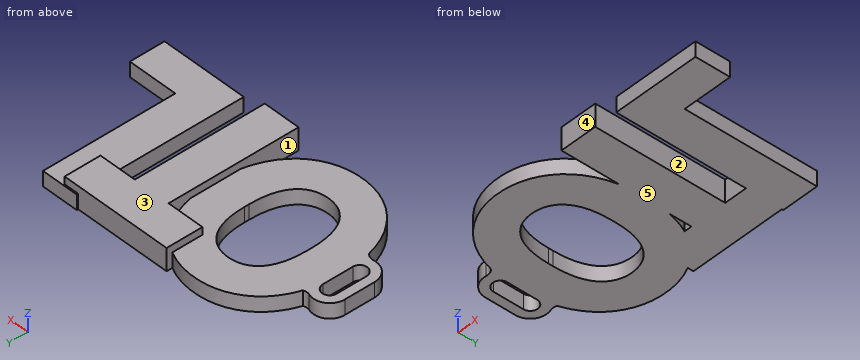
from build123d import *

# Parameters (mm, degrees)
PAD_DEPTH    = 2
PAD001_DEPTH = 3
PAD002_DEPTH = 2
PAD003_DEPTH = 2


with BuildPart() as part:
    # Sketch001 → Pad (new body)
    with BuildSketch(Plane.XY):
        with BuildLine():
            add(Edge.make_bspline(
                [(11.345455, -0.198864), (16.382955, -0.198864), (20.826136, 3.529545), (20.826136, 10.782955)],
                knots=[0, 0, 0, 0, 1, 1, 1, 1], degree=3))
            Line((20.826136, 10.782955), (20.826136, 11.417045))
            add(Edge.make_bspline(
                [(20.826136, 11.417045), (20.826136, 18.670455), (16.382955, 22.4), (11.345455, 22.4)],
                knots=[0, 0, 0, 0, 1, 1, 1, 1], degree=3))
            add(Edge.make_bspline(
                [(11.345455, 22.4), (6.306818, 22.4), (1.903409, 18.670455), (1.903409, 11.417045)],
                knots=[0, 0, 0, 0, 1, 1, 1, 1], degree=3))
            Line((1.903409, 11.417045), (1.903409, 10.782955))
            add(Edge.make_bspline(
                [(1.903409, 10.782955), (1.903409, 3.529545), (6.306818, -0.198864), (11.345455, -0.198864)],
                knots=[0, 0, 0, 0, 1, 1, 1, 1], degree=3))
        make_face()
        with BuildLine():
            add(Edge.make_bspline(
                [(11.345455, 4.363636), (9.004545, 4.363636), (6.782955, 5.948864), (6.782955, 10.782955)],
                knots=[0, 0, 0, 0, 1, 1, 1, 1], degree=3))
            Line((6.782955, 10.782955), (6.782955, 11.417045))
            add(Edge.make_bspline(
                [(6.782955, 11.417045), (6.782955, 16.252273), (9.004545, 17.8375), (11.345455, 17.8375)],
                knots=[0, 0, 0, 0, 1, 1, 1, 1], degree=3))
            add(Edge.make_bspline(
                [(11.345455, 17.8375), (13.685227, 17.8375), (15.946591, 16.252273), (15.946591, 11.417045)],
                knots=[0, 0, 0, 0, 1, 1, 1, 1], degree=3))
            Line((15.946591, 11.417045), (15.946591, 10.782955))
            add(Edge.make_bspline(
                [(15.946591, 10.782955), (15.946591, 5.948864), (13.685227, 4.363636), (11.345455, 4.363636)],
                knots=[0, 0, 0, 0, 1, 1, 1, 1], degree=3))
        make_face(mode=Mode.SUBTRACT)
    extrude(amount=PAD_DEPTH)

    # Sketch003 → Pad001 (join)
    with BuildSketch(Plane(origin=(-7.7, 0, 0), x_dir=(1, 0, 0), z_dir=(0, 0, 1))):
        Polygon((38.234091, 22.181818), (23.278409, 22.181818), (23.278409, 17.381818), (28.2375, 17.381818), (28.2375, -0.034091), (33.196591, -0.034091), (33.196591, 17.381818), (38.234091, 17.381818), align=None)
    extrude(amount=PAD001_DEPTH)

    # Sketch004 → Pad002 (join)
    with BuildSketch(Plane(origin=(-13, 0, 0), x_dir=(1, 0, 0), z_dir=(0, 0, 1))):
        Polygon((46.498864, 4.640909), (46.498864, 22.372727), (41.539773, 22.372727), (41.539773, 0), (53.163636, 0), (53.163636, 4.640909), align=None)
    extrude(amount=PAD002_DEPTH)

    # Sketch005 → Pad003 (join)
    with BuildSketch(Plane(origin=(0.5, 0, 0), x_dir=(1, 0, 0), z_dir=(0, 0, 1))):
        with BuildLine():
            ThreePointArc((-1.797468, 9.715848), (-1.062216, 8.07435), (0.652091, 7.530048))
            ThreePointArc((1.82363, 7.152552), (1.285914, 7.490432), (0.652091, 7.530048))
            Line((1.82363, 7.152552), (2.602532, 9.715848))
            Line((2.602532, 9.715848), (2.602532, 13.715848))
            Line((2.04395, 15.821661), (2.602532, 13.715848))
            ThreePointArc((1.204151, 15.764606), (1.628824, 15.722862), (2.04395, 15.821661))
            ThreePointArc((1.204151, 15.764606), (-0.837718, 15.532928), (-1.797468, 13.715848))
            Line((-1.797468, 13.715848), (-1.797468, 9.715848))
        make_face()
        with BuildLine():
            ThreePointArc((1.402532, 13.715848), (0.402532, 14.715848), (-0.597468, 13.715848))
            Line((-0.597468, 13.715848), (-0.597468, 9.715848))
            ThreePointArc((-0.597468, 9.715848), (0.402532, 8.715848), (1.402532, 9.715848))
            Line((1.402532, 9.715848), (1.402532, 13.715848))
        make_face(mode=Mode.SUBTRACT)
    extrude(amount=PAD003_DEPTH)


solid = part.part
Build history of the part. All positions in model axes, mm. Face numbers are marked on the shaded views. A direction names the side the tool comes from. Coordinates: 2 decimals unless noted, no trailing zeros. Order: outer loops, then holes, each group sorted by start corner. A loop starts at its lowest first (then second) coordinate and runs counter-clockwise, first axis right, second up. Notation, with made-up numbers: (25, 5.25) - (42, 5.25) arc R15 ccw to (42, 9.25) - close; hole circle Ø4 at (58, -22). An arc over 180 degrees is marked (long way). Write each question's results on one line, items separated by ' | '. Start each with the question number.
Item 1: Band-saw the part on A-A on x = 29. Write the cut outline in (y, z).
Item 2: Tool access for the marked faces 4 and 5: list every direction of +Z, -Z, +X, -X, +Y, -Y with a clear straight run to the whole face (end or side of a thin tool).
Item 3: Flat gauge pins, fed straight in: pin 1 (0.5 mm diameter, centred on y = 11, z = 0.5, fed in from +X); pin 2 (11 mm diameter, centred on x = 10.5, y = 12, fed in from +Z); pin 3 (1.6 mm diameter, centred on x = 30.5, z = 1, fed in from +Y); pin 4 (10 mm diameter, centred on x = 35.5, y = 10.5, fed in from -Z). Where does each tip first touch, or does it go through?
Item 4: Wall check: probe 1 along X at (y, z) = (10.5, 1.35); probe 2 along X at (y, z) = (17, 1.05) (1 decimal); probe 3 along X at (y, z) = (8, 0.75). Give the ranges that are in metal, low to high. Write a range as [from, to].
Item 5: Band-saw the part on B-B on y = 3.75. State how many separate pieces and enclosed holes the cut face has, and give its area (3 significant figures).
Item 6: Mould opens along X. For the marked faces 1, 2 and 3 say: released by +X, released by -X, zero draft, split by the parting line, or undercut.
Numbers:
1) outline: (0, 0) - (22.37, 0) - (22.37, 2) - (22.18, 2) - (22.18, 3) - (17.38, 3) - (17.38, 2) - (0, 2) - close
2) face 4: +Z, -Z, +X, -Y | face 5: -Z, +X, -X, +Y, -Y
3) pin 1: x = 33.5 | pin 2: z = 2 | pin 3: y = 22.37 | pin 4: z = 0
4) probe 1: [-1.3, -0.1], [1.9, 6.79], [15.94, 25.5], [28.54, 33.5] | probe 2: [3, 8.8], [13.9, 19.7], [20.5, 25.5], [28.5, 33.5] | probe 3: [-0.47, 7.09], [15.63, 25.5], [28.54, 33.5]
5) separate pieces: 3 | enclosed holes: 0 | area: 68.4 mm^2
6) face 1: undercut | face 2: undercut | face 3: zero draft
